Source: CAD feature listing. Evaluate the final solid. Frame: model axes, mm. Face numbers are marked on the shaded views. A direction names the side the tool comes from. Give positions to 0.01 mm unless a question says otherwise; leave off trailing zeros. Write each loop counter-clockwise with the first axis right and the second up, starting at its lowest first coordinate (ties: lowest second). Pieces come first, ordered by that corner, then holes. Notation, with made-up numbers: M 19,61.5 L 74,61.5 A18 cw 74,88.5 Z; hole C 62.25,43.25 d7. An arc over 180 degrees is marked long. Return JSON: item names as keys, results as strings.
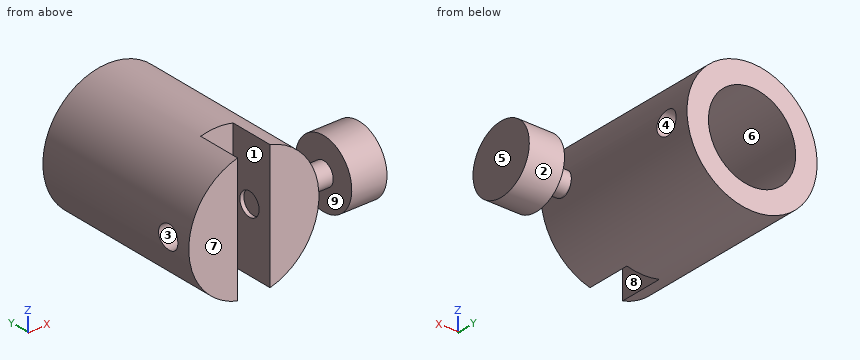
```python
from build123d import *

# Parameters (mm, degrees)
SKETCH1_R               = 9.4742
BOSS_EXTRUDE1_DEPTH     = 25.4
SKETCH2_R               = 6.35
CUT_EXTRUDE1_DEPTH      = 15.9766
CUT_EXTRUDE2_DEPTH      = 29.717258422
CUT_EXTRUDE2_DEPTH_BACK = 29.717258422
CUT_EXTRUDE3_DEPTH      = 29.717258422
CUT_EXTRUDE3_DEPTH_BACK = 29.717258422
SKETCH4_R               = 1.6764
SKETCH5_R               = 1.6764
CUT_EXTRUDE4_DEPTH      = 29.717258577
SKETCH6_R               = 1.6764
BOSS_EXTRUDE2_DEPTH     = 3.683
SKETCH7_R               = 4.9022
BOSS_EXTRUDE3_DEPTH     = 5.1308
SKETCH8_R               = 1.6764
BOSS_EXTRUDE4_DEPTH     = 6.5278


with BuildPart() as part:
    # Sketch1 → Boss-Extrude1 (new body)
    with BuildSketch(Plane(origin=(0, 0, 0), x_dir=(1, 0, 0), z_dir=(0, 1, 0))):
        with Locations(Location((0, 0, 0), (0, 0, 270))):
            Circle(SKETCH1_R)
    extrude(amount=BOSS_EXTRUDE1_DEPTH)

    # Sketch2 → Cut-Extrude1 (cut)
    with BuildSketch(Plane(origin=(0, 25.4, 0), x_dir=(1, 0, 0), z_dir=(0, 1, 0))):
        with Locations(Location((0, 0, 0), (0, 0, 270))):
            Circle(SKETCH2_R)
    extrude(amount=-CUT_EXTRUDE1_DEPTH, mode=Mode.SUBTRACT)

    # Sketch3 → Cut-Extrude2 (cut, two sides: drawn at the far end of the back side and taken through both)
    with BuildSketch(Plane.XY.offset(-CUT_EXTRUDE2_DEPTH_BACK)):
        Polygon((0, 0), (2.3622, 0), (2.3622, 6.4262), (-2.3622, 6.4262), (-2.3622, 0), align=None)
    extrude(amount=CUT_EXTRUDE2_DEPTH + CUT_EXTRUDE2_DEPTH_BACK, mode=Mode.SUBTRACT)

    # Sketch4 → Cut-Extrude3 (cut, two sides: drawn at the far end of the back side and taken through both)
    with BuildSketch(Plane(origin=(0, 0, 0), x_dir=(0, 0, -1), z_dir=(1, 0, 0)).offset(-CUT_EXTRUDE3_DEPTH_BACK)):
        with Locations((0, 3.5814)):
            Circle(SKETCH4_R)
    extrude(amount=CUT_EXTRUDE3_DEPTH + CUT_EXTRUDE3_DEPTH_BACK, mode=Mode.SUBTRACT)

    # Sketch5 → Cut-Extrude4 (cut, through all)
    with BuildSketch(Plane(origin=(0, 0, 0), x_dir=(0, 0, -1), z_dir=(1, 0, 0))):
        with Locations(Location((0, 21.8186, 0), (0, 0, 180))):
            Circle(SKETCH5_R)
    extrude(amount=CUT_EXTRUDE4_DEPTH, mode=Mode.SUBTRACT)



with BuildPart() as body_2:
    # Sketch6 → Boss-Extrude2 (new body)
    with BuildSketch(Plane(origin=(9.4742, 0, 0), x_dir=(0, 0, -1), z_dir=(1, 0, 0))):
        with Locations((0, 3.5814)):
            Circle(SKETCH6_R)
    extrude(amount=BOSS_EXTRUDE2_DEPTH)

    # Sketch7 → Boss-Extrude3 (add)
    with BuildSketch(Plane(origin=(13.1572, 0, 0), x_dir=(0, 0, -1), z_dir=(1, 0, 0))):
        with Locations((0, 3.5814)):
            Circle(SKETCH7_R)
    extrude(amount=BOSS_EXTRUDE3_DEPTH)


with BuildPart() as part_1:
    add(part.part)

    add(body_2.part)  # Boss-Extrude4 merges body 2
    # Sketch8 → Boss-Extrude4 (add)
    with BuildSketch(Plane(origin=(9.4742, 0, 0), x_dir=(0, 0, -1), z_dir=(1, 0, 0))):
        with Locations((0, 3.5814)):
            Circle(SKETCH8_R)
    extrude(amount=-BOSS_EXTRUDE4_DEPTH)


solid = part_1.part
```
1) Cut plane B-B, the plane y = 16. Return the cut outline in (x, z), then the cut area to 3 significant figures.
Numbers:
{"outline": "C 0,0 d18.95; hole C 0,0 d12.7", "area": "155 mm²"}
2) Draft query along Y for the marked faces 1, 2, 3 and 4. Return one class per face: released by +Y, released by -Y, zero draft, split by the parting line, or undercut.
Numbers:
{"face 1": "zero draft", "face 2": "split by the parting line", "face 3": "undercut", "face 4": "undercut"}
3) Cut plane C-C, the plane z = 3. Return the cut outline in (x, y).
Numbers:
{"outline": "M -8.99,0 L -2.36,0 L -2.36,6.43 L 2.36,6.43 L 2.36,0 L 8.99,0 L 8.99,25.4 L 5.6,25.4 L 5.6,9.42 L -5.6,9.42 L -5.6,25.4 L -8.99,25.4 Z; M 13.16,-0.3 L 18.29,-0.3 L 18.29,7.46 L 13.16,7.46 Z"}
4) Cut plane D-D, the plane x = -3.5. Return the cut outline in (y, z), then the cut area to 3 significant figures.
Numbers:
{"outline": "M 0,-8.8 L 25.4,-8.8 L 25.4,-5.3 L 9.42,-5.3 L 9.42,5.3 L 25.4,5.3 L 25.4,8.8 L 0,8.8 Z; hole C 3.58,0 d3.35", "area": "269 mm²"}
5) Cut plane A-A, the plane x = 0. Return the cut outline in (y, z).
Numbers:
{"outline": "M 6.43,-9.47 L 25.4,-9.47 L 25.4,-6.35 L 9.42,-6.35 L 9.42,6.35 L 25.4,6.35 L 25.4,9.47 L 6.43,9.47 Z"}
6) Set-up query: the marked faces 5, 6, 7, 8 and 9. Return all of +Z, -Z, +X, -X, +Y, -Y with unobstructed straight access to the full face (end or side cutting, diameter ignored); none if empty.
Numbers:
{"face 5": "+Z, -Z, +X, +Y, -Y", "face 6": "+Y", "face 7": "+Z, -Z, -X, -Y", "face 8": "+Z, -Z, -Y", "face 9": "none"}
7) Line query: line 1 (Y direction, x = 8.3, z = 0) (3 decimals); line 2 (X direction, y = 3.75, z = -2.75); line 3 (Y direction, x = -7.25, z = 0) (3 decimals). Output: solid intervals per line, ascending. Write a range as [from, to].
Numbers:
{"line 1": "y = [0, 20.142], [23.495, 25.4]", "line 2": "x = [-9.07, -2.36], [2.36, 9.07], [13.16, 18.29]", "line 3": "y = [0, 1.905], [5.258, 25.4]"}
8) Contact query for flat-ended pins moving along their axis: pin 1 Ø3 at (y, z) = (4.5, 1) entering from -X; pin 2 Ø5.5 at (x, z) = (5, 1.5) entering from -Y; pin 3 Ø2 at (x, z) = (15, 5.5) entering from -Y; pin 4 Ø2 at (x, y) = (-1.5, 11) entering from +Z. Output: stop coordinate, or through.
Numbers:
{"pin 1": "stops at x = -9.47", "pin 2": "stops at y = 0", "pin 3": "stops at y = 1.64", "pin 4": "stops at z = 9.46"}
